Design review of the part built by this model. Coordinates are the model's own, in mm. A direction names the side the tool comes from. Coordinates: 2 decimals unless noted, no trailing zeros. Loops run counter-clockwise (first coordinate to the right, second up) from the corner with the lowest first, then second, coordinate; pieces in that order, holes last. Notation, with made-up numbers: (20.5, 31) -> (57.5, 31) arc R23 ccw to (57.5, 59) -> close; hole circle Ø2 at (3.25, 17.5). An arc over 180 degrees is marked (long way). Use a Markdown table: item, result. Add a question column.
Q1. Clearance check with flat-ended pins moving along their axes: pin 1 Ø4 at (x, z) = (36.5, 1) entering from -Y; pin 2 Ø3.5 at (x, y) = (40.04, 6.55) entering from +Z; pin 3 Ø6.5 at (x, y) = (40.04, 6.55) entering from +Z; pin 4 Ø1 at (x, z) = (41.5, 2.5) entering from +Y. State where each tip first meets the part, or that it passes through.
Q2. Take a section at D-D on x = 32. Write out the cut boundary in (y, z), plus the area to 3 significant figures.
Q3. Take a section at A-A on y = 7.5. Write out the cut boundary in (x, z).
Q4. Take a section at C-C on x = 39. Write out the cut boundary in (y, z).
Q5. For probe 1 along X at (y, z) = (6.5, 4.25); probe 2 along X at (y, z) = (6.75, 2.25); probe 3 along Y at (x, z) = (36.5, 6), list the stretches that pass through material, from the lowest coordinate up.
Q6. Draft analysis for pull direction X (two halves, no side actions). For faces 3 (the face through (22.08, 0.76, 3.74)), 4 (the face through (23.46, 6.72, 5.35)), 5 (the face through (32.71, 9.51, 5.35)), 6 (the face through (23, 7, 7.595)), state which applies: pulls with the +X half, pulls with the -X half, needs draft (parallel to the pull), parting line crosses it, or undercut.
Q7. Take a section at B-B on z = 6.5. Write out the cut boundary in (x, y), plus the area to 3 significant figures.
Q8. For faces 1 (the face through (32.61, 3.62, 5.35)), 2 (the face through (3.214, 5.775, 3.744)), list the 3-axis set-ups (+Z, -Z, +X, -X, +Y, -Y) from which the entire face can be reached by the end or side of a thin tool; tool diameter is ignored.
Solid Edge part; units mm, degrees
sketch "Sketch1" plane through (0, 0, 0) normal (0, 0, -1) x (-1, 0, 0)
  circle A0 centre (-5.091, 6.5528) radius 2.032
  circle A1 centre (-40.0411, 6.5528) radius 2.1806
  line L0 (-39.7635, 13.0959) -> (-4.8761, 11.6154)
  line L1 (-4.8761, 1.4902) -> (-39.7635, 0.0097)
  arc A2 (-39.7635, 0.0097) -> (-39.7635, 13.0959) centre (-40.0411, 6.5528) cw
  arc A3 (-4.8761, 11.6154) -> (-4.8761, 1.4902) centre (-5.091, 6.5528) cw
extrude "Protrusion1" add sketch "Sketch1" against normal blind 7.5946
sketch "Sketch2" plane through (23.307, 6.5528, 7.5946) normal (0, 0, 1) x (-0.9991, -0.0424, 0)
  line L0 (-16.1522, 4.3971) -> (-1.9834, 2.2188)
  arc A0 (-2.3772, -2.0855) -> (-1.9834, 2.2188) centre (-2.3124, 0.0788) ccw
  line L1 (-16.4741, -3.0134) -> (-2.3772, -2.0855)
  arc A1 (-16.4741, -3.0134) -> (-16.1522, 4.3971) centre (-16.7191, 0.7095) cw
extrude "Enlèvement_matière_1" cut sketch "Sketch2" against normal blind 4.5466
properties part number "AC_1.08"
Answer list:
| question | item | result |
|---|---|---|
| 1 | pin 1 | y = 0.06 |
| 1 | pin 2 | through |
| 1 | pin 3 | z = 3.05 |
| 1 | pin 4 | y = 13.03 |
| 2 | outline | (0.34, 0) -> (12.77, 0) -> (12.77, 7.59) -> (9.43, 7.59) -> (9.43, 3.05) -> (3.69, 3.05) -> (3.69, 7.59) -> (0.34, 7.59) -> close |
| 2 | area | 68.3 mm² |
| 3 | outline | (0.11, 0) -> (3.29, 0) -> (3.29, 7.59) -> (0.11, 7.59) -> close; (6.89, 0) -> (38.08, 0) -> (38.08, 3.05) -> (23.66, 3.05) -> (23.66, 7.59) -> (6.89, 7.59) -> close; (42.01, 0) -> (46.52, 0) -> (46.52, 7.59) -> (43.65, 7.59) -> (43.65, 3.05) -> (42.01, 3.05) -> close |
| 4 | outline | (0.04, 0) -> (4.64, 0) -> (4.64, 3.05) -> (2.91, 3.05) -> (2.91, 7.59) -> (0.04, 7.59) -> close; (8.47, 0) -> (13.06, 0) -> (13.06, 7.59) -> (10.19, 7.59) -> (10.19, 3.05) -> (8.47, 3.05) -> close |
| 5 | probe 1 | 0.02 to 3.06, 7.12 to 23.46, 43.77 to 46.59 |
| 5 | probe 2 | 0.03 to 3.07, 7.11 to 37.87, 42.21 to 46.59 |
| 5 | probe 3 | 0.15 to 3.19, 9.92 to 12.96 |
| 6 | face 3 | pulls with the -X half |
| 6 | face 4 | undercut |
| 6 | face 5 | undercut |
| 6 | face 6 | needs draft |
| 7 | outline | (4.88, 1.49) -> (39.76, 0.01) arc R6.55 ccw (long way) to (39.76, 13.1) -> (4.88, 11.62) arc R5.07 ccw to start; hole circle Ø4.06 at (5.09, 6.55); hole (25.38, 4.42) -> (39.63, 2.84) arc R3.73 ccw (long way) to (39.64, 10.26) -> (25.59, 8.74) arc R2.17 ccw to start |
| 7 | area | 386 mm² |
| 8 | face 1 | +Z |
| 8 | face 2 | +Z, -Z |
